```python
from build123d import *

# Parameters (mm, degrees)
SKETCH1_W           = 130
SKETCH1_H           = 84
BOSS_EXTRUDE1_DEPTH = 2
SKETCH2_R           = 2
CUT_EXTRUDE1_DEPTH  = 2
CUT_EXTRUDE2_DEPTH  = 2


with BuildPart() as part:
    # Sketch1 → Boss-Extrude1 (new body)
    with BuildSketch(Plane.XY):
        Rectangle(SKETCH1_W, SKETCH1_H)
    extrude(amount=BOSS_EXTRUDE1_DEPTH)

    # Sketch2 → Cut-Extrude1 (cut)
    with BuildSketch(Plane.XY.offset(2)):
        with Locations((55, -30)):
            Circle(SKETCH2_R)
        with Locations((-55, -30)):
            Circle(SKETCH2_R)
        with Locations((55, 30)):
            Circle(SKETCH2_R)
        with Locations((-5, 30)):
            Circle(SKETCH2_R)
    extrude(amount=-CUT_EXTRUDE1_DEPTH, mode=Mode.SUBTRACT)

    # Sketch3 → Cut-Extrude2 (cut)
    with BuildSketch(Plane.XY.offset(2)):
        with BuildLine():
            Line((-55, 32), (-31.229864945, 32))
            ThreePointArc((-31.229864945, 32), (-29.229864945, 30), (-31.229864945, 28))
            Line((-31.229864945, 28), (-55, 28))
            ThreePointArc((-55, 28), (-57, 30), (-55, 32))
        make_face()
    extrude(amount=-CUT_EXTRUDE2_DEPTH, mode=Mode.SUBTRACT)


solid = part.part
```
Check sheet for the modelled part. Datum: model origin and axes. Units: mm. Coordinates: 2 decimals unless noted, no trailing zeros. Order: outer loops, then holes, each group sorted by start corner. A loop starts at its lowest first (then second) coordinate and runs counter-clockwise, first axis right, second up. Notation, with made-up numbers: (83, 52) -> (101, 52) arc R17 cw to (101, 58) -> close; hole circle Ø8 at (58, 34). An arc over 180 degrees is marked (long way). Write item = value, one per line. Start each with the question number.
1) Cross-section at C-C (x = 55). Enter the section's corners in (y, z).
2) Cross-section at A-A (y = -30). Enter the section's corners in (x, z), then the cut area to 3 significant figures.
3) Cross-section at B-B (x = -5). Enter the section's corners in (y, z).
4) Go/stop test with a flat-tipped pin: P1, Ø2.5, axis at x = -55, y = -30, coming from the -Z side. Record where the tip stops, or that it passes through.
5) Material ranges on L1, parallel to Y at x = 55, z = 0.9; L2, parallel to Y at x = -5, z = 0.95; L3, parallel to Y at x = 54.5, z = 1.25, recorded low to high.
6) Mould release check, pull along X, two halves, no side actions. Record for faces 1 (the flat face through (-1, 1, 2)), 2 (the cylindrical face through (-5, 28, 1)): +X half, -X half, draft (parallel to the pull), parting line (faces both ways), or undercut.
Ans:
q1.outline = (-42, 0) -> (-32, 0) -> (-32, 2) -> (-42, 2) -> close; (-28, 0) -> (28, 0) -> (28, 2) -> (-28, 2) -> close; (32, 0) -> (42, 0) -> (42, 2) -> (32, 2) -> close
q2.outline = (-65, 0) -> (-57, 0) -> (-57, 2) -> (-65, 2) -> close; (-53, 0) -> (53, 0) -> (53, 2) -> (-53, 2) -> close; (57, 0) -> (65, 0) -> (65, 2) -> (57, 2) -> close
q2.area = 244 mm²
q3.outline = (-42, 0) -> (28, 0) -> (28, 2) -> (-42, 2) -> close; (32, 0) -> (42, 0) -> (42, 2) -> (32, 2) -> close
q4.P1 = through
q5.L1 = -42 to -32, -28 to 28, 32 to 42
q5.L2 = -42 to 28, 32 to 42
q5.L3 = -42 to -31.94, -28.06 to 28.06, 31.94 to 42
q6.face_1 = draft
q6.face_2 = undercut
